Geometry: see drawing. Coordinates: mm, zero at the bounding-box minimum. Coordinates: 2 decimals unless noted, no trailing zeros. Order: outer loops, then holes, each group sorted by start corner. A loop starts at its lowest first (then second) coordinate and runs counter-clockwise, first axis right, second up.
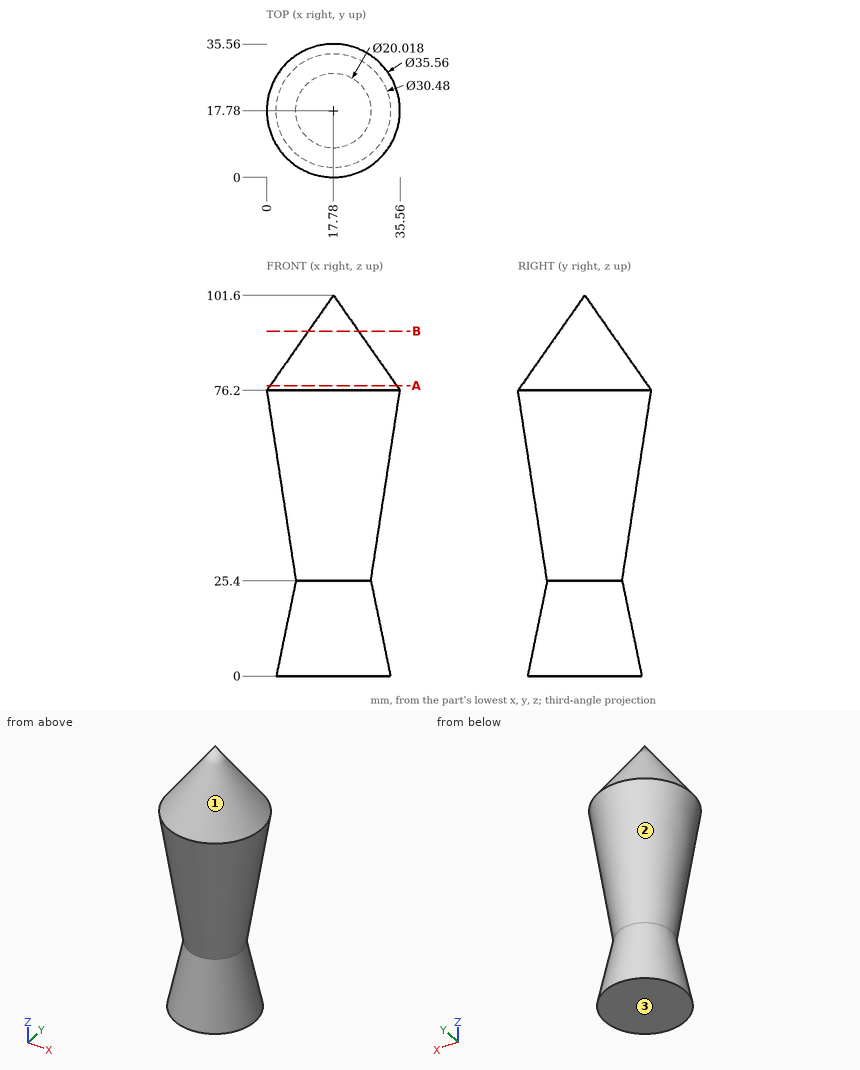
Q1. Section query A-A on z = 77.5. Output: boundary loops of the cut face in (x, y).
Solutions:
outline: circle Ø33.74 at (17.78, 17.78)
Q2. Pin query (flat end, axial travel): P1, Ø4, axis at x = 11, z = 15.5, coming from the +Y side; P2, Ø2, axis at y = 11.5, z = 79, coming from the -X side; P3, Ø12, axis at x = 16.5, z = 88.5, coming from the +Y side. Return the tip coordinate at first contact, or that it passes through.
Solutions:
P1: stops at y = 28.95
P2: stops at x = 2.4
P3: stops at y = 31.11
Q3. Pull-direction query (Z, two-part tool) for the marked faces 1, 2 and 3; classes: pulls with the +Z half, pulls with the -Z half, needs draft (parallel to the pull), parting line crosses it, or undercut.
Solutions:
face 1: pulls with the +Z half
face 2: undercut
face 3: pulls with the -Z half
Q4. Section query B-B on z = 92. Output: boundary loops of the cut face in (x, y), plus the area to 3 significant figures.
Solutions:
outline: circle Ø13.44 at (17.78, 17.78)
area: 142 mm2
Q5. Material intervals for line 1 along X through (y, z) = (13, 26.5) (3 decimals); line 2 along X through (y, z) = (17, 63.5); line 3 along Y through (x, z) = (9.5, 9), sorted ascending.
Solutions:
line 1: x = 8.795 to 26.765
line 2: x = 1.96 to 33.6
line 3: y = 7.26 to 28.3
